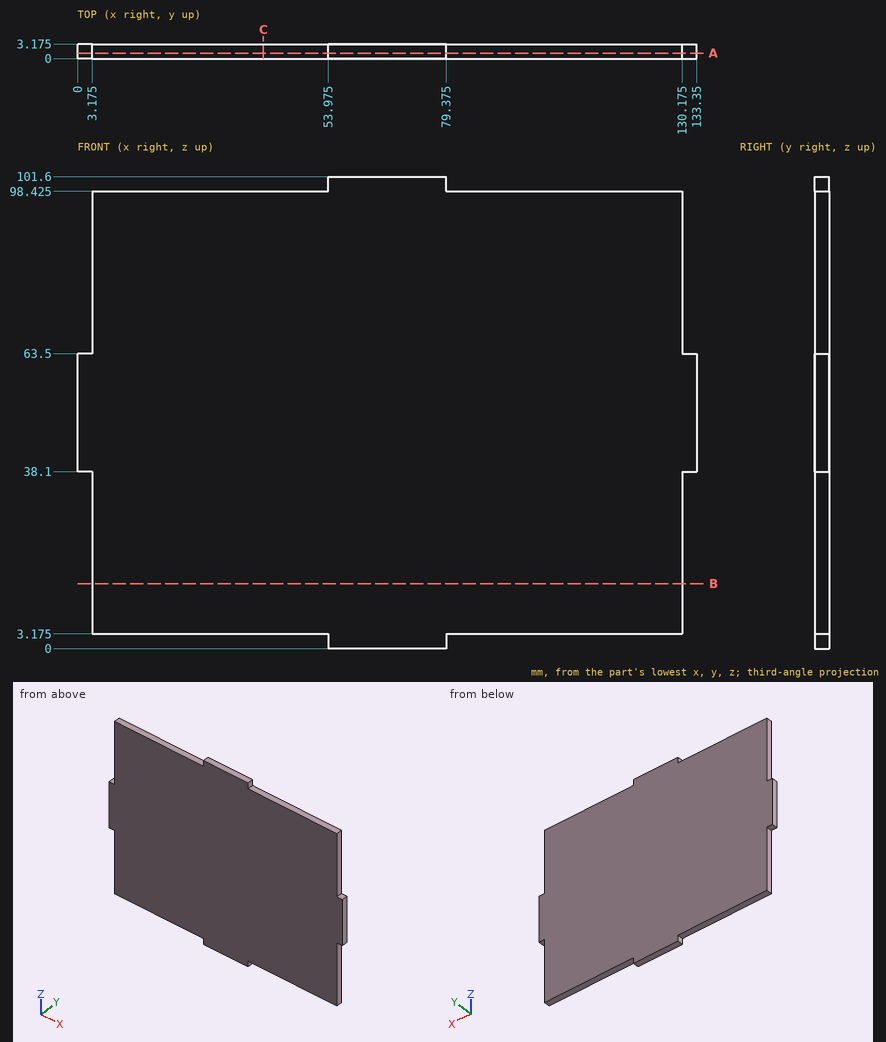
Part print with two shaded views. Sizes in mm from the minimum x, y, z corner. Coordinates: 2 decimals unless noted, no trailing zeros. Order: outer loops, then holes, each group sorted by start corner. A loop starts at its lowest first (then second) coordinate and runs counter-clockwise, first axis right, second up. Notation, with made-up numbers: (35, 82.25) - (41, 82.25) arc R22 cw to (41, 110.25) - close; hole circle Ø4 at (43.25, -18). An arc over 180 degrees is marked (long way). Write item = value, one per line. Start each with the question number.
1) Flat gauge pins, fed straight in: pin 1 Ø1.6 at (y, z) = (1, 100.5) entering from +X (3 decimals); pin 2 Ø1.5 at (x, y) = (52, 1) entering from -Z (3 decimals); pin 3 Ø1 at (y, z) = (2, 78.5) entering from -X (3 decimals). Where does each tip first touch, or does it go through?
2) Saw through at A-A on y = 1.2. Write the cut outline in (x, z) (3 decimals), then the cut area to 3 significant figures.
3) Saw through at C-C on x = 40. Write the cut outline in (y, z) (3 decimals).
4) Saw through at B-B on z = 14. Write the cut outline in (x, y) (3 decimals).
5) Wall check: line 1 along Z through (x, y) = (89.5, 1.8) (3 decimals); line 2 along X through (y, z) = (0.9, 32.5) (3 decimals). Give the ranges that are in metal, low to high. Write a range as from..to.
From the geometry:
q1.pin_1 = 79.375
q1.pin_2 = 3.175
q1.pin_3 = 3.175
q2.outline = (0, 38.1) - (3.175, 38.1) - (3.175, 3.175) - (53.975, 3.175) - (53.975, 0) - (79.375, 0) - (79.375, 3.175) - (130.175, 3.175) - (130.175, 38.1) - (133.35, 38.1) - (133.35, 63.5) - (130.175, 63.5) - (130.175, 98.425) - (79.375, 98.425) - (79.375, 101.6) - (53.975, 101.6) - (53.975, 98.425) - (3.175, 98.425) - (3.175, 63.5) - (0, 63.5) - close
q2.area = 12,400 mm^2
q3.outline = (0, 3.175) - (3.175, 3.175) - (3.175, 98.425) - (0, 98.425) - close
q4.outline = (3.175, 0) - (130.175, 0) - (130.175, 3.175) - (3.175, 3.175) - close
q5.line_1 = 3.175..98.425
q5.line_2 = 3.175..130.175
